Source: CAD feature listing. Evaluate the final solid. Frame: model axes, mm. Round coordinates to 2 decimals unless told otherwise and drop trailing zeros. Loops run counter-clockwise (first coordinate to the right, second up) from the corner with the lowest first, then second, coordinate; pieces in that order, holes last.
(1) Section D-D, the plane y = 27.5. Return the cut outline in (x, z).
(2) Section C-C, the plane x = 68.5. Return the cut outline in (y, z), plus the area to 3 significant figures.
(3) Material intervals for probe 1 along Y at (x, z) = (121, 23); probe 2 along Z at (x, y) = (74, 24.5); probe 3 along Y at (x, z) = (81, 2.25), sorted ascending.
(4) First-contact query: pin 1 Ø1.5 at (x, y) = (114.5, 34.5) entering from -Z; pin 2 Ø4 at (x, y) = (92.5, 31) entering from +Z. Flat tips, straight axial feed; report the tip coordinate or a pass-through.
(5) Mould query, pull axis Z, two halves, no side actions, for faces 1 (the cylindrical face through (90.41, 1, 17.07)), 2 (the cylindrical face through (77.267, 0.942, 0.993)), 3 (the flat face through (77, 2.032, 14)), 4 (the cylindrical face through (142.13, 1, 18.51)). Classes: pulls with the +Z half, pulls with the -Z half, needs draft (parallel to the pull), parting line crosses it, or undercut.
(6) Section B-B, the plane z = 8. Return the cut outline in (x, y), plus the area to 3 significant figures.
(7) Section A-A, the plane x = 25.4. Return the cut outline in (y, z).
Autodesk Inventor part; units mm, degrees
ref_plane "YZ Plane" through (0, 0, 0) normal (1, 0, 0) x (0, 1, 0)
ref_plane "XZ Plane" through (0, 0, 0) normal (0, 1, 0) x (-1, 0, 0)
ref_plane "XY Plane" through (0, 0, 0) normal (0, 0, 1) x (1, 0, 0)
sketch "Sketch1" plane through (0, 0, 0) normal (0, 0, 1) x (1, 0, 0)
  line L0 (0, 0) -> (152.4, 0)
  line L1 (152.4, 0) -> (152.4, 46.736)
  line L2 (152.4, 46.736) -> (0, 46.736)
  line L3 (0, 46.736) -> (0, 0)
  dimension "d0" = 152.4
  dimension "d1" = 46.736
extrude "Plate1" add sketch "Sketch1" along normal blind 2.032
sketch "Sketch2" plane through (0, 44.704, 0) normal (0, 1, 0) x (-1, 0, 0)
  line L0 (-152.4, 0) -> (0, 0)
  line L1 (0, 0) -> (0, 24.13)
  line L2 (0, 24.13) -> (-152.4, 24.13)
  line L3 (-152.4, 24.13) -> (-152.4, 0)
edge flange "Flange1" height 24.13 angle 90 thickness 2.032 bend radius 1.27 thickness toward (0, 1, 0) relief tear relief width 2.032 relief depth 1.016 edges at (76.2, 46.736, 2.032) wall of the first edge with corners at (152.4, 44.704, 0) (0, 44.704, 0) (0, 44.704, 24.13) (152.4, 44.704, 24.13)
bend "Bend1"
corner "Corner1"
sketch "Sketch3" plane through (152.4, 2.032, 0) normal (0, -1, 0) x (1, 0, 0)
  line L0 (-152.4, 0) -> (0, 0)
  line L1 (0, 0) -> (0, 24.13)
  line L2 (0, 24.13) -> (-152.4, 24.13)
  line L3 (-152.4, 24.13) -> (-152.4, 0)
edge flange "Flange2" height 24.13 angle 90 thickness 2.032 bend radius 1.27 thickness toward (0, -1, 0) relief tear relief width 2.032 relief depth 1.016 edges at (76.2, 0, 2.032) wall of the first edge with corners at (0, 2.032, 0) (152.4, 2.032, 0) (152.4, 2.032, 24.13) (0, 2.032, 24.13)
bend "Bend2"
corner "Corner2"
sketch "Sketch4" plane through (0, 46.736, 24.13) normal (0, 1, 0) x (1, 0, 0)
  line L0 (0, 0) -> (0, 20.828)
  line L1 (0, 24.13) -> (152.4, 24.13)
  point P0 (12.7, 5.08)
  dimension "d23" = 12.7
  dimension "d24" = 19.05
hole "Hole1" at (12.7, 46.736, 19.05) direction (0, -1, 0) diameter 4.9784 end through all
pattern_linear "Rectangular Pattern1" count 11 spacing 12.7 along (1, 0, 0) of "Hole1"
sketch "Sketch5" plane through (0, 0, 0) normal (0, 0, -1) x (-1, 0, 0)
  line L0 (-152.4, 3.302) -> (-152.4, 43.434)
  point P0 (0, 0)
  point P1 (-95.25, 23.368)
  point P2 (-152.4, 23.368)
  dimension "d35" = 57.15
hole "Hole2" at (95.25, 23.368, 0) direction (0, 0, 1) diameter 15.875 end through all
equation "\"d30\" = Thickness"
equation "\"d41\" = Thickness"
equation "\"d2\" = Thickness"
equation "\"d3\" = BendReliefWidth"
equation "\"d4\" = BendReliefDepth"
equation "\"d5\" = MinimumRemnant"
equation "\"d6\" = TransitionRadius"
equation "\"d9\" = BendRadius"
equation "\"d10\" = CornerReliefSize"
equation "\"d11\" = GapSize"
equation "\"d12\" = JacobiRadiusSize"
equation "\"d13\" = BendReliefWidth"
equation "\"d14\" = BendReliefDepth"
equation "\"d15\" = MinimumRemnant"
equation "\"d16\" = TransitionRadius"
equation "\"d19\" = BendRadius"
equation "\"d20\" = CornerReliefSize"
equation "\"d21\" = GapSize"
equation "\"d22\" = JacobiRadiusSize"
equation "\"BendReliefWidth\" = Thickness"
equation "\"BendReliefDepth\" = 0.5 * Thickness"
equation "\"CornerReliefSize\" = 4 * Thickness"
equation "\"MinimumRemnant\" = 2 * Thickness"
equation "\"TransitionRadius\" = BendRadius"
equation "\"JacobiRadiusSize\" = BendRadius"
equation "\"GapSize\" = Thickness"
properties part number "Side arm inner" material "Aluminum 6061"
Output values:
1. outline: (0, 0) - (88.47, 0) - (88.47, 2.03) - (0, 2.03) - close; (102.03, 0) - (152.4, 0) - (152.4, 2.03) - (102.03, 2.03) - close
2. outline: (0, 3.3) arc R3.3 ccw to (3.3, 0) - (43.43, 0) arc R3.3 ccw to (46.74, 3.3) - (46.74, 24.13) - (44.7, 24.13) - (44.7, 3.3) arc R1.27 cw to (43.43, 2.03) - (3.3, 2.03) arc R1.27 cw to (2.03, 3.3) - (2.03, 24.13) - (0, 24.13) - close
2. area: 181 mm2
3. probe 1: y = 0 to 2.03, 44.7 to 46.74
3. probe 2: z = 0 to 2.03
3. probe 3: y = 0.17 to 2.59, 44.15 to 46.56
4. pin 1: stops at z = 0
4. pin 2: stops at z = 2.03
5. face 1: undercut
5. face 2: pulls with the -Z half
5. face 3: needs draft
5. face 4: undercut
6. outline: (0, 0) - (152.4, 0) - (152.4, 2.03) - (0, 2.03) - close; (0, 44.7) - (152.4, 44.7) - (152.4, 46.74) - (0, 46.74) - close
6. area: 619 mm2
7. outline: (0, 3.3) arc R3.3 ccw to (3.3, 0) - (43.43, 0) arc R3.3 ccw to (46.74, 3.3) - (46.74, 16.56) - (44.7, 16.56) - (44.7, 3.3) arc R1.27 cw to (43.43, 2.03) - (3.3, 2.03) arc R1.27 cw to (2.03, 3.3) - (2.03, 16.56) - (0, 16.56) - close; (0, 21.54) - (2.03, 21.54) - (2.03, 24.13) - (0, 24.13) - close; (44.7, 21.54) - (46.74, 21.54) - (46.74, 24.13) - (44.7, 24.13) - close
